Can you work these out from the model? Positions are in its coordinate system, mm. A direction names the side the tool comes from. Give positions to 0.01 mm unless a question says otherwise; leave off trailing zeros. Write each loop counter-clockwise with the first axis right and the second up, starting at its lowest first coordinate (ties: lowest second). Pieces come first, ordered by that corner, then holes.
from build123d import *

# Parameters (mm, degrees)
SKETCH1_R                       = 38.1
BOSS_EXTRUDE1_DEPTH             = 6.35
SKETCH2_R                       = 19.05
BOSS_EXTRUDE2_DEPTH             = 19.05
SKETCH3_R                       = 16.0782
CUT_EXTRUDE1_DEPTH              = 60.56828015
CUT_EXTRUDE2_REACH              = 61.568
SKETCH4_R                       = 2.978668017
SKETCH5_R                       = 23.8633
SKETCH5_R_2                     = 21.7297
CUT_EXTRUDE3_DEPTH              = 1.3208
FILLET1_R                       = 0.127
FILLET2_R                       = 0.254
SKETCH6_R                       = 16.0782
CUT_EXTRUDE4_DEPTH              = 60.56828015
TAP_DRILL_FOR_1_4_20_TAP1_D     = 5.1054
TAP_DRILL_FOR_1_4_20_TAP1_DEPTH = 6.35


with BuildPart() as part:
    # Sketch1 → Boss-Extrude1 (new body)
    with BuildSketch(Plane.XY):
        Circle(SKETCH1_R)
    boss_extrude1 = extrude(amount=BOSS_EXTRUDE1_DEPTH)

    # Sketch2 → Boss-Extrude2 (add)
    with BuildSketch(Plane.XY.offset(6.35)):
        with Locations(Location((0, 0, 0), (0, 0, 180))):
            Circle(SKETCH2_R)
    extrude(amount=BOSS_EXTRUDE2_DEPTH)

    # Sketch3 → Cut-Extrude1 (cut, through all)
    with BuildSketch(Plane.XY.offset(25.4)):
        Circle(SKETCH3_R)
    extrude(amount=-CUT_EXTRUDE1_DEPTH, mode=Mode.SUBTRACT)

    # Sketch4 → Cut-Extrude2 (cut, up to next)
    with BuildSketch(Plane.XY, mode=Mode.PRIVATE) as cut_extrude2_sk1:
        with Locations(Location((0, 31.75, 0), (0, 0, 180))):
            Circle(SKETCH4_R)
    cut_extrude2_tool1 = extrude(cut_extrude2_sk1.sketch, amount=CUT_EXTRUDE2_REACH, mode=Mode.PRIVATE) & part.part
    # Sketch4 → Cut-Extrude2 (cut, up to next)
    with BuildSketch(Plane.XY, mode=Mode.PRIVATE) as cut_extrude2_sk2:
        with Locations(Location((27.49630657, 15.875, 0), (0, 0, 180))):
            Circle(SKETCH4_R)
    cut_extrude2_tool2 = extrude(cut_extrude2_sk2.sketch, amount=CUT_EXTRUDE2_REACH, mode=Mode.PRIVATE) & part.part
    # Sketch4 → Cut-Extrude2 (cut, up to next)
    with BuildSketch(Plane.XY, mode=Mode.PRIVATE) as cut_extrude2_sk3:
        with Locations(Location((27.49630657, -15.875, 0), (0, 0, 180))):
            Circle(SKETCH4_R)
    cut_extrude2_tool3 = extrude(cut_extrude2_sk3.sketch, amount=CUT_EXTRUDE2_REACH, mode=Mode.PRIVATE) & part.part
    # Sketch4 → Cut-Extrude2 (cut, up to next)
    with BuildSketch(Plane.XY, mode=Mode.PRIVATE) as cut_extrude2_sk4:
        with Locations(Location((0, -31.75, 0), (0, 0, 180))):
            Circle(SKETCH4_R)
    cut_extrude2_tool4 = extrude(cut_extrude2_sk4.sketch, amount=CUT_EXTRUDE2_REACH, mode=Mode.PRIVATE) & part.part
    # Sketch4 → Cut-Extrude2 (cut, up to next)
    with BuildSketch(Plane.XY, mode=Mode.PRIVATE) as cut_extrude2_sk5:
        with Locations(Location((-27.49630657, -15.875, 0), (0, 0, 180))):
            Circle(SKETCH4_R)
    cut_extrude2_tool5 = extrude(cut_extrude2_sk5.sketch, amount=CUT_EXTRUDE2_REACH, mode=Mode.PRIVATE) & part.part
    # Sketch4 → Cut-Extrude2 (cut, up to next)
    with BuildSketch(Plane.XY, mode=Mode.PRIVATE) as cut_extrude2_sk6:
        with Locations(Location((-27.49630657, 15.875, 0), (0, 0, 180))):
            Circle(SKETCH4_R)
    cut_extrude2_tool6 = extrude(cut_extrude2_sk6.sketch, amount=CUT_EXTRUDE2_REACH, mode=Mode.PRIVATE) & part.part
    add(cut_extrude2_tool1.solids().sort_by_distance((0, 31.75, 0))[0], mode=Mode.SUBTRACT)
    add(cut_extrude2_tool2.solids().sort_by_distance((27.496307, 15.875, 0))[0], mode=Mode.SUBTRACT)
    add(cut_extrude2_tool3.solids().sort_by_distance((27.496307, -15.875, 0))[0], mode=Mode.SUBTRACT)
    add(cut_extrude2_tool4.solids().sort_by_distance((0, -31.75, 0))[0], mode=Mode.SUBTRACT)
    add(cut_extrude2_tool5.solids().sort_by_distance((-27.496307, -15.875, 0))[0], mode=Mode.SUBTRACT)
    add(cut_extrude2_tool6.solids().sort_by_distance((-27.496307, 15.875, 0))[0], mode=Mode.SUBTRACT)

    # Sketch5 → Cut-Extrude3 (cut)
    with BuildSketch(Plane(origin=(0, 0, 0), x_dir=(-1, 0, 0), z_dir=(0, 0, -1))):
        Circle(SKETCH5_R)
        Circle(SKETCH5_R_2, mode=Mode.SUBTRACT)
    extrude(amount=-CUT_EXTRUDE3_DEPTH, mode=Mode.SUBTRACT)

    # Fillet1
    fillet1_edges = [part.edges().sort_by_distance(p)[0] for p in [
        (23.8633, 0, 0),
        (21.7297, 0, 0),
    ]]
    fillet(fillet1_edges, radius=FILLET1_R)

    # Fillet2
    fillet2_edges = [part.edges().sort_by_distance(p)[0] for p in [
        (23.8633, 0, 1.3208),
        (21.7297, 0, 1.3208),
    ]]
    fillet(fillet2_edges, radius=FILLET2_R)

    # Mirror1: Boss-Extrude1 across plane
    add(boss_extrude1.mirror(Plane.XY.offset(15.875)))

    # Sketch6 → Cut-Extrude4 (cut, through all)
    with BuildSketch(Plane(origin=(0, 0, 25.4), x_dir=(-1, 0, 0), z_dir=(0, 0, -1))):
        with Locations(Location((0, 0, 0), (0, 0, 180))):
            Circle(SKETCH6_R)
    extrude(amount=-CUT_EXTRUDE4_DEPTH, mode=Mode.SUBTRACT)

    # Tap Drill for 1/4-20 Tap1
    with Locations(Plane(origin=(0, 31.75, 31.75), x_dir=(1, 0, 0), z_dir=(0, 0, 1))):
        with Locations((0, 0), (31.75, -31.75), (0, -63.5), (-31.75, -31.75)):
            Hole(TAP_DRILL_FOR_1_4_20_TAP1_D / 2, depth=TAP_DRILL_FOR_1_4_20_TAP1_DEPTH)


solid = part.part
(1) Will these pins go through, and if not, where does the flat tip stop? P1, Ø4, axis at y = 17, z = 5, coming from the -X side; P2, Ø4, axis at y = 7, z = 26, coming from the +X side; P3, Ø4, axis at y = 19, z = 16, coming from the -X side.
Returned:
P1: stops at x = -35.02
P2: stops at x = 37.77
P3: stops at x = -8.6
(2) Imagine slicing it at D-D, the plane x = -31.75. Write out the boundary of the cut face in (y, z), plus the area to 3 significant figures.
Returned:
outline: (-21.06, 0) - (21.06, 0) - (21.06, 6.35) - (-21.06, 6.35) - close; (-21.06, 25.4) - (-2.55, 25.4) - (-2.55, 31.75) - (-21.06, 31.75) - close; (2.55, 25.4) - (21.06, 25.4) - (21.06, 31.75) - (2.55, 31.75) - close
area: 503 mm2
(3) For faces 1 (the face through (25, 1, 0)), 2 (the face through (29.86, 17.69, 3.13)), 3 (the face through (29.315, 0.767, 28.531)), which set-ups out of +Z, -Z, +X, -X, +Y, -Y let a thin tool reach every point of the face, with its end or its side?
Returned:
face 1: -Z, +X, -X, +Y, -Y
face 2: -Z
face 3: +Z
(4) Imagine slicing it at A-A, the plane x = 0. Give the number of separate pieces and of enclosed holes in the cut face, plus the area to 3 significant figures.
Returned:
separate pieces: 6
enclosed holes: 0
area: 526 mm2
(5) Imagine slicing it at C-C, the plane z = 28.5. Write out the boundary of the cut face in (x, y), plus the area to 3 significant figures.
Returned:
outline: circle Ø76.2 at (0, 0); hole circle Ø5.11 at (-31.75, 0); hole circle Ø32.16 at (0, 0); hole circle Ø5.11 at (0, -31.75); hole circle Ø5.11 at (0, 31.75); hole circle Ø5.11 at (31.75, 0)
area: 3,670 mm2
(6) If I drill on L1, parallel to Y at x = 0, z = 28; L2, parallel to Y at x = 0, z = 3.25; L3, parallel to Z at x = 30, y = 5, over which ranges is the centre line in solid material (lowest first)?
Returned:
L1: y = -38.1 to -34.3, -29.2 to -16.08, 16.08 to 29.2, 34.3 to 38.1
L2: y = -38.1 to -34.73, -28.77 to -16.08, 16.08 to 28.77, 34.73 to 38.1
L3: z = 0 to 6.35, 25.4 to 31.75
(7) If we mould it in two halves opening along X, with no side actions, what happens to faces 4 (the face through (7, -21, 1.321)), 5 (the face through (-30.235, -23.183, 28.619)), 6 (the face through (7.9, 17.5, 6.35))? For each: +X half, -X half, draft (parallel to the pull), parting line (faces both ways), or undercut.
Returned:
face 4: undercut
face 5: parting line
face 6: draft
